```python
from build123d import *

# Parameters (mm, degrees)
BOSS_EXTRUDE1_DEPTH     = 12.7
BACKREST_BRACKET_SLOT_W = 12.7
BACKREST_BRACKET_SLOT_H = 8.89
CUT_EXTRUDE3_DEPTH      = 12.7
BACKREST_SCREW_HOLE_R   = 1.397
CUT_EXTRUDE4_DEPTH      = 6.35
CUT_EXTRUDE5_DEPTH      = 25.4
BOSS_EXTRUDE2_DEPTH     = 3.175
SKETCH37_W              = 12.7
SKETCH37_H              = 101.6
CUT_EXTRUDE7_DEPTH      = 8.89
SKETCH38_R              = 3.175
CUT_EXTRUDE8_DEPTH      = 12.7
SKETCH39_W              = 12.7
SKETCH39_H              = 12.7
CUT_EXTRUDE9_DEPTH      = 8.89
CUT_EXTRUDE10_START     = -12.7
SKETCH40_R              = 1.397
CUT_EXTRUDE10_DEPTH     = 6.35


with BuildPart() as part:
    # Main Body → Boss-Extrude1 (new body)
    with BuildSketch(Plane(origin=(0, 0, 0), x_dir=(1, 0, 0), z_dir=(0, 1, 0))):
        with BuildLine():
            Line((-317.5, -107.95), (-317.5, 107.95))
            ThreePointArc((-317.5, 107.95), (-311.920384182, 121.420384182), (-298.45, 127))
            Line((-298.45, 127), (298.45, 127))
            ThreePointArc((298.45, 127), (311.920384182, 121.420384182), (317.5, 107.95))
            Line((317.5, 107.95), (317.5, -107.95))
            ThreePointArc((317.5, -107.95), (311.920384182, -121.420384182), (298.45, -127))
            Line((298.45, -127), (-298.45, -127))
            ThreePointArc((-298.45, -127), (-311.920384182, -121.420384182), (-317.5, -107.95))
        make_face()
    extrude(amount=BOSS_EXTRUDE1_DEPTH)

    # Backrest Bracket Slot → Cut-Extrude3 (cut)
    with BuildSketch(Plane.XY.offset(127)):
        with Locations((-292.1, 8.255)):
            Rectangle(BACKREST_BRACKET_SLOT_W, BACKREST_BRACKET_SLOT_H)
    cut_extrude3 = extrude(amount=-CUT_EXTRUDE3_DEPTH, mode=Mode.SUBTRACT)

    # Backrest Screw Hole → Cut-Extrude4 (cut)
    with BuildSketch(Plane.XY.offset(114.3)):
        with Locations((-292.1, 8.255)):
            Circle(BACKREST_SCREW_HOLE_R)
    cut_extrude4 = extrude(amount=-CUT_EXTRUDE4_DEPTH, mode=Mode.SUBTRACT)

    # Mirror1: Cut-Extrude3, Cut-Extrude4 across plane
    add(cut_extrude3.mirror(Plane.XY), mode=Mode.SUBTRACT)
    add(cut_extrude4.mirror(Plane.XY), mode=Mode.SUBTRACT)

    # Couch Foot Slits → Cut-Extrude5 (cut)
    with BuildSketch(Plane(origin=(0, 12.7, 0), x_dir=(1, 0, 0), z_dir=(0, 1, 0))):
        with BuildLine():
            Line((-247.65, 101.6), (-184.15, 101.6))
            Line((-184.15, 101.6), (-184.15, 50.8))
            Line((-184.15, 50.8), (-247.65, 50.8))
            ThreePointArc((-247.65, 50.8), (-256.630256121, 54.519743879), (-260.35, 63.5))
            Line((-260.35, 63.5), (-260.35, 88.9))
            ThreePointArc((-260.35, 88.9), (-256.630256121, 97.880256121), (-247.65, 101.6))
        make_face()
        with BuildLine():
            Line((292.1, 88.9), (292.1, 63.5))
            ThreePointArc((292.1, 63.5), (288.380256121, 54.519743879), (279.4, 50.8))
            Line((279.4, 50.8), (215.9, 50.8))
            Line((215.9, 50.8), (215.9, 101.6))
            Line((215.9, 101.6), (279.4, 101.6))
            ThreePointArc((279.4, 101.6), (288.380256121, 97.880256121), (292.1, 88.9))
        make_face()
        with BuildLine():
            Line((-247.65, -50.8), (-184.15, -50.8))
            Line((-184.15, -50.8), (-184.15, -101.6))
            Line((-184.15, -101.6), (-247.65, -101.6))
            ThreePointArc((-247.65, -101.6), (-256.630256121, -97.880256121), (-260.35, -88.9))
            Line((-260.35, -88.9), (-260.35, -63.5))
            ThreePointArc((-260.35, -63.5), (-256.630256121, -54.519743879), (-247.65, -50.8))
        make_face()
        with BuildLine():
            Line((292.1, -63.5), (292.1, -88.9))
            ThreePointArc((292.1, -88.9), (288.380256121, -97.880256121), (279.4, -101.6))
            Line((279.4, -101.6), (215.9, -101.6))
            Line((215.9, -101.6), (215.9, -50.8))
            Line((215.9, -50.8), (279.4, -50.8))
            ThreePointArc((279.4, -50.8), (288.380256121, -54.519743879), (292.1, -63.5))
        make_face()
    extrude(amount=-CUT_EXTRUDE5_DEPTH, mode=Mode.SUBTRACT)

    # Sketch24 → Boss-Extrude2 (add, symmetric)
    with BuildSketch(Plane(origin=(0, 6.35, 0), x_dir=(1, 0, 0), z_dir=(0, 1, 0))):
        with BuildLine():
            Line((-15.24, -133.35), (10.16, -133.35))
            ThreePointArc((10.16, -133.35), (14.650128061, -131.490128061), (16.51, -127))
            Line((16.51, -127), (19.05, -127))
            ThreePointArc((19.05, -127), (16.446179285, -133.286179285), (10.16, -135.89))
            Line((10.16, -135.89), (-15.24, -135.89))
            ThreePointArc((-15.24, -135.89), (-21.526179285, -133.286179285), (-24.13, -127))
            Line((-24.13, -127), (-21.59, -127))
            ThreePointArc((-21.59, -127), (-19.730128061, -131.490128061), (-15.24, -133.35))
        make_face()
        with BuildLine():
            Line((-257.81, -133.35), (-232.41, -133.35))
            ThreePointArc((-232.41, -133.35), (-227.919871939, -131.490128061), (-226.06, -127))
            Line((-226.06, -127), (-223.52, -127))
            ThreePointArc((-223.52, -127), (-226.123820715, -133.286179285), (-232.41, -135.89))
            Line((-232.41, -135.89), (-257.81, -135.89))
            ThreePointArc((-257.81, -135.89), (-264.096179285, -133.286179285), (-266.7, -127))
            Line((-266.7, -127), (-264.16, -127))
            ThreePointArc((-264.16, -127), (-262.300128061, -131.490128061), (-257.81, -133.35))
        make_face()
        with BuildLine():
            Line((227.33, -133.35), (252.73, -133.35))
            ThreePointArc((252.73, -133.35), (257.220128061, -131.490128061), (259.08, -127))
            Line((259.08, -127), (261.62, -127))
            ThreePointArc((261.62, -127), (259.016179285, -133.286179285), (252.73, -135.89))
            Line((252.73, -135.89), (227.33, -135.89))
            ThreePointArc((227.33, -135.89), (221.043820715, -133.286179285), (218.44, -127))
            Line((218.44, -127), (220.98, -127))
            ThreePointArc((220.98, -127), (222.839871939, -131.490128061), (227.33, -133.35))
        make_face()
    boss_extrude2 = extrude(amount=BOSS_EXTRUDE2_DEPTH, both=True)

    # Mirror2: Boss-Extrude2 across plane
    add(boss_extrude2.mirror(Plane.XY))

    # Sketch37 → Cut-Extrude7 (cut)
    with BuildSketch(Plane(origin=(0, 12.7, 0), x_dir=(1, 0, 0), z_dir=(0, 1, 0))):
        with Locations((-292.1, 0)):
            Rectangle(SKETCH37_W, SKETCH37_H)
    extrude(amount=-CUT_EXTRUDE7_DEPTH, mode=Mode.SUBTRACT)

    # Sketch38 → Cut-Extrude8 (cut)
    with BuildSketch(Plane(origin=(0, 12.7, 0), x_dir=(1, 0, 0), z_dir=(0, 1, 0))):
        with Locations((-245.11, -114.3)):
            Circle(SKETCH38_R)
        with Locations((-2.54, -114.3)):
            Circle(SKETCH38_R)
        with Locations((240.03, -114.3)):
            Circle(SKETCH38_R)
    cut_extrude8 = extrude(amount=-CUT_EXTRUDE8_DEPTH, mode=Mode.SUBTRACT)

    # Mirror3: Cut-Extrude8 across plane
    add(cut_extrude8.mirror(Plane.XY), mode=Mode.SUBTRACT)

    # Sketch39 → Cut-Extrude9 (cut)
    with BuildSketch(Plane(origin=(0, 12.7, 0), x_dir=(1, 0, 0), z_dir=(0, 1, 0))):
        with Locations((-292.1, -95.25)):
            Rectangle(SKETCH39_W, SKETCH39_H)
    cut_extrude9 = extrude(amount=-CUT_EXTRUDE9_DEPTH, mode=Mode.SUBTRACT)

    # Sketch40 → Cut-Extrude10 (cut)
    with BuildSketch(Plane.XY.offset(114.3).offset(CUT_EXTRUDE10_START)):
        with Locations((-292.1, 8.255)):
            Circle(SKETCH40_R)
    cut_extrude10 = extrude(amount=CUT_EXTRUDE10_DEPTH, mode=Mode.SUBTRACT)

    # Mirror5: Cut-Extrude9, Cut-Extrude10 across plane
    add(cut_extrude9.mirror(Plane.XY), mode=Mode.SUBTRACT)
    add(cut_extrude10.mirror(Plane.XY), mode=Mode.SUBTRACT)


solid = part.part
```
CAD build for the part. Positions are in the model's coordinates, mm. A direction names the side the tool comes from. Round coordinates to 2 decimals unless told otherwise and drop trailing zeros. Order: outer loops, then holes, each group sorted by start corner. A loop starts at its lowest first (then second) coordinate and runs counter-clockwise, first axis right, second up.
Q1. Wall check: L1, parallel to Z at x = 228.5, y = 12; L2, parallel to Z at x = -2.54, y = 5.75 (3 decimals); L3, parallel to X at y = 2.5, z = -74. Give the ranges that are in metal, low to high.
Q2. Two-plate mould, pull along X, no slides. Class faces 1 (the cylindrical face through (311.77, 6.26, -121.57)), 2 (the cylindrical face through (-312.07, 6.26, -121.27)), 3 (the flat face through (247, 6, -101.6)): pulls with the +X half, pulls with the -X half, needs draft (parallel to the pull), parting line crosses it, or undercut.
Q3. Slice it at B-B (x = 188.5). Write the cut outline in (y, z).
Q4. Slice it at A-A (z = 95). Write the cut outline in (x, y), and give its area (3 significant figures).
Q5. Drop flat-ended pins along their axis: pin 1 (2.5 mm diameter, centred on x = -249, z = 133, fed in from +Y) (3 decimals); pin 2 (7 mm diameter, centred on y = 6.5, z = 120, fed in from -X); pin 3 (5 mm diameter, centred on x = 164, y = 11, fed in from +Z). Give the stop position or say it passes through.
Q6. Which spindle directions (+Z, -Z, +X, -X, +Y, -Y) get a long thin tool onto all of the face, cutting with end or side? Do faces 4 (the flat face through (-292, 3.81, -1)), 5 (the cylindrical face through (-256.73, 6.44, 54.62)), 6 (the cylindrical face through (-311.77, 6.26, 121.57)). Say none if no direction does.
Results below:
1. L1: z = -127 to -101.6, -50.8 to 50.8, 101.6 to 127
1. L2: z = -135.89 to -133.35, -127 to -117.475, -111.125 to 111.125, 117.475 to 127, 133.35 to 135.89
1. L3: x = -317.5 to -260.35, -184.15 to 215.9, 292.1 to 317.5
2. face 1: pulls with the +X half
2. face 2: pulls with the -X half
2. face 3: undercut
3. outline: (0, -127) - (12.7, -127) - (12.7, 127) - (0, 127) - close
4. outline: (-317.5, 0) - (-258.79, 0) - (-258.79, 12.7) - (-285.75, 12.7) - (-285.75, 3.81) - (-298.45, 3.81) - (-298.45, 12.7) - (-317.5, 12.7) - close; (-184.15, 0) - (215.9, 0) - (215.9, 12.7) - (-184.15, 12.7) - close; (290.54, 0) - (317.5, 0) - (317.5, 12.7) - (290.54, 12.7) - close
4. area: 6,060 mm2
5. pin 1: stops at y = 9.525
5. pin 2: stops at x = -315.47
5. pin 3: stops at z = 127
6. face 4: +Y
6. face 5: +Y, -Y
6. face 6: +Z, -X, +Y, -Y
